```python
from build123d import *

# Parameters (mm, degrees)
F1_DEPTH    = 12.7
F2_W        = 29.4221741813
F2_H        = 3.8190931082
F3_DEPTH    = 25.4
F4_T1_DEPTH = 58.42
F4_T3_DEPTH = 41.9312775373
F4_T5_DEPTH = 42.0824239574


# Not quite as in the source:
# - a fillet or chamfer that OpenCascade refuses, or shapes differently, is made with other operations: its cross-section is extruded or revolved along the edge and cut away or added


with BuildPart() as f1:
    # F0 (on Front) → F1 (new body)
    with BuildSketch(Plane.XZ):
        Polygon((6.3818255705, 18.0452149361), (-26.6381744295, 18.0452149361), (-26.6381744295, 2.3869331926), (6.3818255705, 2.3869331926), (6.3818255705, 10.2160740644), align=None)
        with BuildLine():
            ThreePointArc((35.8039997518, 10.2160740644), (21.6048326678, 16.0544570681), (6.3818255705, 18.0452149361))
            Line((6.3818255705, 18.0452149361), (6.3818255705, 10.2160740644))
            Line((6.3818255705, 10.2160740644), (35.8039997518, 10.2160740644))
        make_face()
    extrude(amount=F1_DEPTH)

    # F2 (on face) → F3 (cut)
    with BuildSketch(Plane(origin=(0, 0, 10.2160740644), x_dir=(1, 0, 0), z_dir=(0, 0, -1))):
        with Locations((21.0929126611, 6.5879346803)):
            Rectangle(F2_W, F2_H)
    extrude(amount=-F3_DEPTH, mode=Mode.SUBTRACT)

    # F4: fillet of radius 5.08 on 4 edges, made by hand

    # F4_s2 → F4_t1 (cut)
    with BuildSketch(Plane.YZ.offset(-39.3381744295)):
        with BuildLine():
            ThreePointArc((-12.7, 7.4669331926), (-11.2121024484, 3.8748307442), (-7.62, 2.3869331926))
            Line((-7.62, 2.3869331926), (-12.7, 2.3869331926))
            Line((-12.7, 2.3869331926), (-12.7, 7.4669331926))
        make_face()
        with BuildLine():
            ThreePointArc((0, 7.4669331926), (-1.4878975516, 3.8748307442), (-5.08, 2.3869331926))
            Line((-5.08, 2.3869331926), (0, 2.3869331926))
            Line((0, 2.3869331926), (0, 7.4669331926))
        make_face()
    extrude(amount=F4_T1_DEPTH, mode=Mode.SUBTRACT)

    # F4_s4 → F4_t3 (cut)
    with BuildSketch(Plane.YZ.offset(6.3818255705)):
        with BuildLine():
            ThreePointArc((-12.7, 15.2197154068), (-11.5099874467, 11.9525457349), (-8.4974812344, 10.2160740644))
            Line((-8.4974812344, 10.2160740644), (-12.7, 10.2160740644))
            Line((-12.7, 10.2160740644), (-12.7, 15.2197154068))
        make_face()
    extrude(amount=F4_T3_DEPTH, mode=Mode.SUBTRACT)

    # F4_s6 → F4_t5 (cut)
    with BuildSketch(Plane.YZ.offset(6.3818255705)):
        with BuildLine():
            ThreePointArc((0, 15.2801739748), (-1.3486069412, 11.8329858685), (-4.6783881262, 10.2160740644))
            Line((-4.6783881262, 10.2160740644), (0, 10.2160740644))
            Line((0, 10.2160740644), (0, 15.2801739748))
        make_face()
    extrude(amount=F4_T5_DEPTH, mode=Mode.SUBTRACT)


solid = f1.part
```
Check sheet for the modelled part. Datum: model origin and axes. Units: mm. A direction names the side the tool comes from. Give positions to 0.01 mm unless a question says otherwise; leave off trailing zeros. Loops run counter-clockwise (first coordinate to the right, second up) from the corner with the lowest first, then second, coordinate; pieces in that order, holes last. Notation, with made-up numbers: (37, 58.5) - (80, 58.5) arc R3 cw to (80, 62.5) - close; hole circle Ø2 at (-34.75, 24.5). An arc over 180 degrees is marked (long way). One line per question, with ' | ' between items. Start each with the question number.
1. Set-up check for faces 5 (the cylindrical face through (-10.359, -1.449, 3.915)), 6 (the cylindrical face through (20.887, -1.313, 11.872)), 7 (the flat face through (18, -4.678, 13)): record each of +Z, -Z, +X, -X, +Y, -Y from which the full face is reachable in a straight line by a thin tool's end or side.
2. Gauge pin test, flat ends, axial feed: pin 1 Ø6 at (y, z) = (-5, 5.5) entering from +X; pin 2 Ø6.5 at (x, z) = (26.5, 16) entering from +Y; pin 3 Ø4 at (x, z) = (16.5, 13) entering from -Y. Record the tip position at first contact, or that the pin passes through.
3. Draft check along Y on faces 1 (the flat face through (6.382, -6, 8)), 2 (the cylindrical face through (20.89, -11.54, 11.99)), 3 (the flat face through (-26.638, -6, 10)), 4 (the flat face through (18, -8.497, 13)). Enter one of: released by +Y, released by -Y, zero draft, split by the parting line, or undercut.
4. Material ranges on line 1 along X through (y, z) = (-3.5, 7.25); line 2 along Y through (x, z) = (30.5, 12); line 3 along Y through (x, z) = (5.5, 7.25), recorded low to high. Write a range as [from, to].
5. Cross-section at C-C, the plane x = 2. Enter the section's corners in (y, z), plus the area to 3 significant figures.
6. Cross-section at B-B, the plane z = 11.75. Enter the section's corners in (x, y), plus the area to 3 significant figures.
7. Cross-section at A-A, the plane x = 15. Enter the section's corners in (y, z).
8. Cross-section at D-D, the plane y = -7. Enter the section's corners in (x, z), plus the area to 3 significant figures.
Check result:
1) face 5: -Z, +X, -X, +Y | face 6: -Z, +X, +Y | face 7: +Z, -Z, +X
2) pin 1: stops at x = 6.38 | pin 2: stops at y = 0 | pin 3: stops at y = -12.7
3) face 1: undercut | face 2: released by -Y | face 3: zero draft | face 4: undercut
4) line 1: x = [-26.64, 6.38] | line 2: y = [-11.55, -8.5], [-4.68, -1.2] | line 3: y = [-12.7, 0]
5) outline: (-12.7, 7.47) arc R5.08 ccw to (-7.62, 2.39) - (-5.08, 2.39) arc R5.08 ccw to (0, 7.47) - (0, 18.05) - (-12.7, 18.05) - close | area: 188 mm2
6) outline: (-26.64, -12.7) - (6.38, -12.7) - (6.38, -11.33) - (32.95, -11.33) - (32.95, -8.5) - (6.38, -8.5) - (6.38, -4.68) - (32.95, -4.68) - (32.95, -1.43) - (6.38, -1.43) - (6.38, 0) - (-26.64, 0) - close | area: 581 mm2
7) outline: (-12.7, 15.22) arc R5.08 ccw to (-8.5, 10.22) - (-8.5, 17.41) - (-12.7, 17.41) - close; (-4.68, 10.22) arc R5.08 ccw to (0, 15.28) - (0, 17.41) - (-4.68, 17.41) - close
8) outline: (-26.64, 2.39) - (6.38, 2.39) - (6.38, 18.05) - (-26.64, 18.05) - close | area: 517 mm2
